Can you work these out from the drawing? Everything is in mm from the part's minimum corner. A direction names the side the tool comes from. Round coordinates to 2 decimals unless told otherwise and drop trailing zeros. Write each loop counter-clockwise with the first axis right and the second up, starting at its lowest first coordinate (ties: lowest second). Pieces come first, ordered by that corner, then holes. Notation, with made-up numbers: (42.5, 85.25) - (74.5, 85.25) arc R8 ccw to (74.5, 97.25) - close; hole circle Ø2 at (-17.75, 76). An arc over 180 degrees is marked (long way). One line per item, written item: value. Start each with the question number.
(1) I want a section at A-A on x = 11. List the corners of the cut face in (y, z) for me, plus the area to 3 significant figures.
(2) Thinking about a two-plate mould opening in Z: for the marked faces 6, 7 and 8, which applies, +Z half, -Z half, draft (parallel to the pull), parting line (faces both ways), or undercut?
(3) If I drill on L1, parallel to X at y = 1.75, z = 5.5; L2, parallel to Y at x = 10.5, z = 6.25; L3, parallel to X at y = 1, z = 5.25, over which ranges is the centre line in solid material (lowest first)? Write a range as from..to.
(4) I want a section at B-B on z = 10.25. List the corners of the cut face in (x, y) for me.
(5) I'm going to push flat-ended pins straight in: pin 1 Ø5.5 at (x, z) = (4.58, 4.64) entering from -Y; pin 2 Ø3 at (y, z) = (12.5, 6) entering from -X; pin 3 Ø3.5 at (y, z) = (18.5, 7) entering from -X. Where does each tip first touch, or does it pass through?
(6) On a 3-axis mill with a long thin cutter (end or side, diameter ignored), from which of +Z, -Z, +X, -X, +Y, -Y can I reach the whole of each face in a straight line? I mean the marked faces 1, 2, 3, 4 and 5. Say none if no direction works.
(7) I want a section at C-C on y = 15.75. List the corners of the cut face in (x, z) for me.
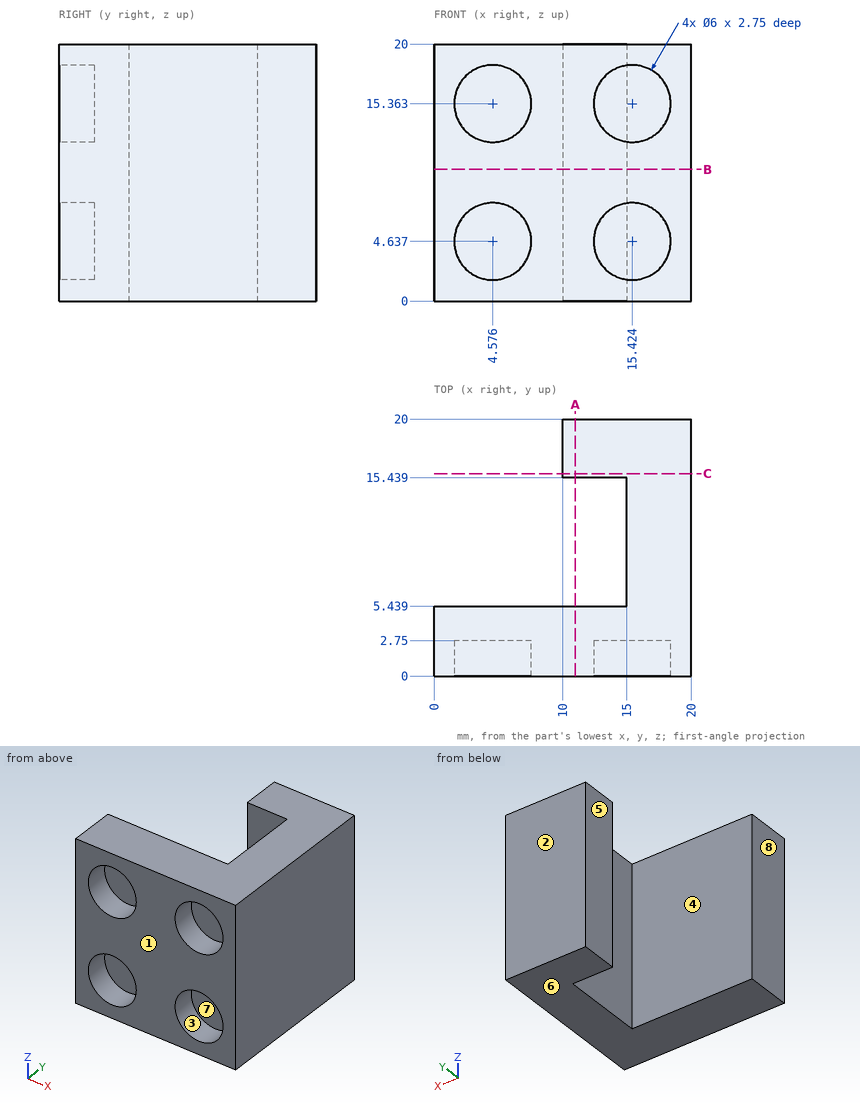
Established:
1. outline: (0, 0) - (5.44, 0) - (5.44, 20) - (0, 20) - close; (15.44, 0) - (20, 0) - (20, 20) - (15.44, 20) - close
1. area: 200 mm2
2. face 6: -Z half
2. face 7: undercut
2. face 8: draft
3. L1: 0..1.7, 7.45..12.55, 18.3..20
3. L2: 0..5.44, 15.44..20
3. L3: 0..1.64, 7.51..12.49, 18.36..20
4. outline: (0, 0) - (20, 0) - (20, 20) - (10, 20) - (10, 15.44) - (15, 15.44) - (15, 5.44) - (0, 5.44) - close
5. pin 1: y = 2.75
5. pin 2: x = 15
5. pin 3: x = 10
6. face 1: +Z, -Z, +X, -X, -Y
6. face 2: +Z, -Z, +X, -X, +Y
6. face 3: -Y
6. face 4: +Z, -Z, -X
6. face 5: +Z, -Z, -X, +Y
7. outline: (10, 0) - (20, 0) - (20, 20) - (10, 20) - close
